from build123d import *

# Parameters (mm, degrees)
SKETCH1_W                = 457.2
SKETCH1_H                = 609.6
BOSS_EXTRUDE1_DEPTH      = 6.35
CUT_EXTRUDE4_DEPTH       = 763.026457874
CUT_EXTRUDE4_DEPTH_BACK  = 763.026457874
SKETCH3_W                = 12.7
SKETCH3_H                = 355.6
CUT_EXTRUDE5_DEPTH       = 763.026457874
CUT_EXTRUDE5_DEPTH_BACK  = 763.026457874
CUT_EXTRUDE7_DEPTH       = 763.026457874
CUT_EXTRUDE7_DEPTH_BACK  = 763.026457874
SKETCH7_W                = 6.35
SKETCH7_H                = 127
CUT_EXTRUDE8_DEPTH       = 763.026457874
CUT_EXTRUDE8_DEPTH_BACK  = 763.026457874
CUT_EXTRUDE10_START      = -6.35
CUT_EXTRUDE10_OUTLINE_W  = 6.35
CUT_EXTRUDE10_OUTLINE_H  = 127
CUT_EXTRUDE10_DEPTH      = 6.35
CUT_EXTRUDE11_DEPTH      = 763.026457874
CUT_EXTRUDE11_DEPTH_BACK = 763.026457874
CUT_EXTRUDE12_DEPTH      = 759.233608461
CUT_EXTRUDE12_DEPTH_BACK = 759.233608461
SKETCH2_R                = 6.604
CUT_EXTRUDE13_DEPTH      = 759.233608461


# Read off the part's stored shape, not the designer's step: Cut-Extrude10
with BuildPart() as part:
    # Sketch1 → Boss-Extrude1 (new body)
    with BuildSketch(Plane(origin=(0, 0, 0), x_dir=(1, 0, 0), z_dir=(0, 1, 0))):
        with Locations((-228.6, 304.8)):
            Rectangle(SKETCH1_W, SKETCH1_H)
    extrude(amount=BOSS_EXTRUDE1_DEPTH)

    # Sketch3 → Cut-Extrude4 (cut, two sides: drawn at the far end of the back side and taken through both)
    with BuildSketch(Plane(origin=(0, 6.35, 0), x_dir=(1, 0, 0), z_dir=(0, 1, 0)).offset(-CUT_EXTRUDE4_DEPTH_BACK)):
        with Locations((-450.85, 304.8)):
            Rectangle(SKETCH3_W, SKETCH3_H)
    extrude(amount=CUT_EXTRUDE4_DEPTH + CUT_EXTRUDE4_DEPTH_BACK, mode=Mode.SUBTRACT)

    # Sketch5 → Cut-Extrude5 (cut, two sides: drawn at the far end of the back side and taken through both)
    with BuildSketch(Plane(origin=(0, 6.35, 0), x_dir=(1, 0, 0), z_dir=(0, 1, 0)).offset(-CUT_EXTRUDE5_DEPTH_BACK)):
        Polygon((1339.563236556, 482.6), (0, 482.6), (-12.7, 482.6), (-12.7, 127), (0, 127), (1339.563236556, 127), (4018.689709667, 127), (4018.689709667, 482.6), align=None)
    extrude(amount=CUT_EXTRUDE5_DEPTH + CUT_EXTRUDE5_DEPTH_BACK, mode=Mode.SUBTRACT)

    # Sketch7 → Cut-Extrude7 (cut, two sides: drawn at the far end of the back side and taken through both)
    with BuildSketch(Plane(origin=(0, 6.35, 0), x_dir=(1, 0, 0), z_dir=(0, 1, 0)).offset(-CUT_EXTRUDE7_DEPTH_BACK)):
        with Locations((-3.175, 63.5)):
            Rectangle(SKETCH7_W, SKETCH7_H)
    extrude(amount=CUT_EXTRUDE7_DEPTH + CUT_EXTRUDE7_DEPTH_BACK, mode=Mode.SUBTRACT)

    # Sketch8 → Cut-Extrude8 (cut, two sides: drawn at the far end of the back side and taken through both)
    with BuildSketch(Plane(origin=(0, 6.35, 0), x_dir=(1, 0, 0), z_dir=(0, 1, 0)).offset(-CUT_EXTRUDE8_DEPTH_BACK)):
        Polygon((-6.35, 2136.014036469), (-6.35, 609.6), (-6.35, 482.6), (-6.35, -1043.814036469), (3046.478072938, -1043.814036469), (3046.478072938, 2136.014036469), align=None)
    extrude(amount=CUT_EXTRUDE8_DEPTH + CUT_EXTRUDE8_DEPTH_BACK, mode=Mode.SUBTRACT)

    # Cut-Extrude10 outline → Cut-Extrude10 (cut)
    with BuildSketch(Plane(origin=(0, 6.35, 0), x_dir=(1, 0, 0), z_dir=(0, 1, 0)).offset(CUT_EXTRUDE10_START)):
        with Locations((-454.025, 546.1)):
            Rectangle(CUT_EXTRUDE10_OUTLINE_W, CUT_EXTRUDE10_OUTLINE_H)
    extrude(amount=CUT_EXTRUDE10_DEPTH, mode=Mode.SUBTRACT)

    # Sketch11 → Cut-Extrude11 (cut, two sides: drawn at the far end of the back side and taken through both)
    with BuildSketch(Plane(origin=(0, 6.35, 0), x_dir=(1, 0, 0), z_dir=(0, 1, 0)).offset(-CUT_EXTRUDE11_DEPTH_BACK)):
        Polygon((-450.85, 1645.896828812), (-450.85, 127), (-450.85, 0), (-450.85, -1518.896828812), (-3488.643657625, -1518.896828812), (-3488.643657625, 1645.896828812), align=None)
    extrude(amount=CUT_EXTRUDE11_DEPTH + CUT_EXTRUDE11_DEPTH_BACK, mode=Mode.SUBTRACT)

    # Sketch6 → Cut-Extrude12 (cut, two sides: drawn at the far end of the back side and taken through both)
    with BuildSketch(Plane(origin=(0, 6.35, 0), x_dir=(1, 0, 0), z_dir=(0, 1, 0)).offset(-CUT_EXTRUDE12_DEPTH_BACK)):
        Polygon((-171.45, -1351.158484296), (-171.45, 0), (-171.45, 6.35), (-285.75, 6.35), (-285.75, 0), (-285.75, -1351.158484296), (-285.75, -4053.475452889), (-171.45, -4053.475452889), align=None)
    extrude(amount=CUT_EXTRUDE12_DEPTH + CUT_EXTRUDE12_DEPTH_BACK, mode=Mode.SUBTRACT)

    # Sketch2 → Cut-Extrude13 (cut, through all)
    with BuildSketch(Plane(origin=(0, 6.35, 0), x_dir=(1, 0, 0), z_dir=(0, 1, 0))):
        with Locations(Location((-292.1, 513.08, 0), (0, 0, 270))):
            Circle(SKETCH2_R)
    extrude(amount=-CUT_EXTRUDE13_DEPTH, mode=Mode.SUBTRACT)


solid = part.part
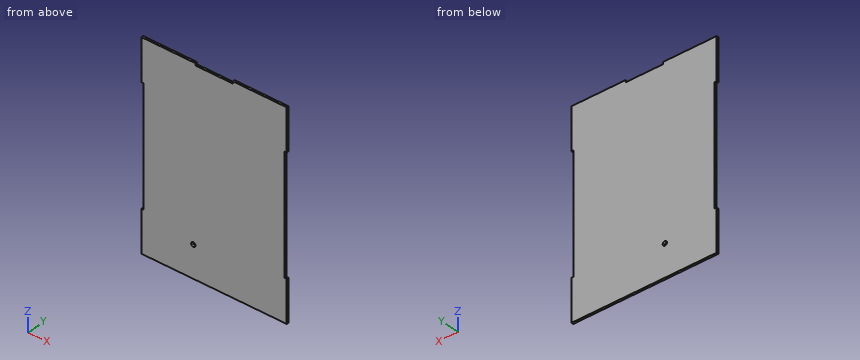
Could you check a few things on this model? Use its own coordinates, in mm. Coordinates: 2 decimals unless noted, no trailing zeros. Loops run counter-clockwise (first coordinate to the right, second up) from the corner with the lowest first, then second, coordinate; pieces in that order, holes last.
1. Imagine slicing it at A-A (x = -292.1). Please give me the cut outline in (y, z).
2. I need wall thicknesses on L1, parallel to Z at x = -292.1, y = 4.5; L2, parallel to X at y = 1.5, z = -513.08; L3, parallel to X at y = 4, z = -344. Which ranges of each line are inside material? Lowest first, please.
3. For P1, Ø2, axis at x = -332, z = -229, coming from the -Y side; P2, Ø3, axis at x = -212, y = 3.5, coming from the +Z side; P3, Ø1.9, axis at y = 2, z = -352, coming from the +X side, each with a flat end and sliding along its axis, tell me the tip position at first contact or that it passes through.
4. Imagine slicing it at D-D (z = -427). Please give me the cut outline in (x, y), and give its area (3 significant figures).
5. Imagine slicing it at B-B (z = -513.08). Please give me the cut outline in (x, y).
6. Imagine slicing it at C-C (y = 2.5). Please give me the cut outline in (x, z).
Computed values:
1. outline: (0, -609.6) - (6.35, -609.6) - (6.35, -519.68) - (0, -519.68) - close; (0, -506.48) - (6.35, -506.48) - (6.35, 0) - (0, 0) - close
2. L1: z = -609.6 to -519.68, -506.48 to 0
2. L2: x = -450.85 to -298.7, -285.5 to -6.35
2. L3: x = -444.5 to -12.7
3. P1: stops at y = 0
3. P2: stops at z = -6.35
3. P3: stops at x = -12.7
4. outline: (-444.5, 0) - (-12.7, 0) - (-12.7, 6.35) - (-444.5, 6.35) - close
4. area: 2,740 mm2
5. outline: (-450.85, 0) - (-298.7, 0) - (-298.7, 6.35) - (-450.85, 6.35) - close; (-285.5, 0) - (-6.35, 0) - (-6.35, 6.35) - (-285.5, 6.35) - close
6. outline: (-450.85, -609.6) - (-6.35, -609.6) - (-6.35, -482.6) - (-12.7, -482.6) - (-12.7, -127) - (-6.35, -127) - (-6.35, 0) - (-171.45, 0) - (-171.45, -6.35) - (-285.75, -6.35) - (-285.75, 0) - (-450.85, 0) - (-450.85, -127) - (-444.5, -127) - (-444.5, -482.6) - (-450.85, -482.6) - close; hole circle Ø13.21 at (-292.1, -513.08)
